Check sheet for the modelled part. Datum: model origin and axes. Units: mm. A direction names the side the tool comes from. Round coordinates to 2 decimals unless told otherwise and drop trailing zeros. Order: outer loops, then holes, each group sorted by start corner. A loop starts at its lowest first (then second) coordinate and runs counter-clockwise, first axis right, second up. Notation, with made-up numbers: (22.25, -40) -> (68.25, -40) arc R22 cw to (68.25, -17) -> close; hole circle Ø11 at (-31.75, 53). An arc over 180 degrees is marked (long way). Use CSV: the item, a comma, the result in double quotes.
```python
from build123d import *

# Parameters (mm, degrees)
BOSS_EXTRUDE1_DEPTH          = 15
SKETCH3_R                    = 40
BOSS_EXTRUDE2_DEPTH          = 100
TAP_DRILL_FOR_M30X2_0_TAP1_D = 28
SKETCH5_R                    = 22.5
CUT_EXTRUDE1_DEPTH           = 50
SKETCH6_W                    = 35
SKETCH6_H                    = 100
BOSS_EXTRUDE3_DEPTH          = 16
SKETCH7_R                    = 15
CUT_EXTRUDE2_DEPTH           = 238.907545067
SKETCH8_W                    = 19
SKETCH8_H                    = 30
SKETCH8_R                    = 5
BOSS_EXTRUDE4_DEPTH          = 77
CUT_EXTRUDE3_DEPTH           = 238.907545067
SKETCH10_R                   = 5
CUT_EXTRUDE4_DEPTH           = 238.907545067
FILLET1_R                    = 1


with BuildPart() as part:
    # Sketch2 → Boss-Extrude1 (new body)
    with BuildSketch(Plane(origin=(0, 0, 0), x_dir=(1, 0, 0), z_dir=(0, 1, 0))):
        with BuildLine():
            Line((-160, 50), (160, 50))
            Line((160, 50), (160, -50))
            Line((160, -50), (-160, -50))
            ThreePointArc((-160, -50), (-210, 0), (-160, 50))
        make_face()
    extrude(amount=BOSS_EXTRUDE1_DEPTH)

    # Sketch3 → Boss-Extrude2 (add)
    with BuildSketch(Plane(origin=(0, 15, 0), x_dir=(1, 0, 0), z_dir=(0, 1, 0))):
        with Locations(Location((-160, 0, 0), (0, 0, 270))):
            Circle(SKETCH3_R)
    extrude(amount=BOSS_EXTRUDE2_DEPTH)

    # Tap Drill for M30x2.0 Tap1 (through all)
    with Locations(Plane(origin=(-160, 115, 0), x_dir=(0, 0, 1), z_dir=(0, 1, 0))):
        with Locations((0, 0)):
            Hole(TAP_DRILL_FOR_M30X2_0_TAP1_D / 2)

    # Sketch5 → Cut-Extrude1 (cut)
    with BuildSketch(Plane(origin=(0, 115, 0), x_dir=(1, 0, 0), z_dir=(0, 1, 0))):
        with Locations(Location((-160, 0, 0), (0, 0, 270))):
            Circle(SKETCH5_R)
    extrude(amount=-CUT_EXTRUDE1_DEPTH, mode=Mode.SUBTRACT)

    # Sketch6 → Boss-Extrude3 (add)
    with BuildSketch(Plane(origin=(0, 15, 0), x_dir=(1, 0, 0), z_dir=(0, 1, 0))):
        with Locations((142.5, 0)):
            Rectangle(SKETCH6_W, SKETCH6_H)
    extrude(amount=BOSS_EXTRUDE3_DEPTH)

    # Sketch7 → Cut-Extrude2 (cut, through all)
    with BuildSketch(Plane(origin=(0, 15, 0), x_dir=(1, 0, 0), z_dir=(0, 1, 0))):
        with Locations(Location((-75, 0, 0), (0, 0, 270))):
            Circle(SKETCH7_R)
    extrude(amount=-CUT_EXTRUDE2_DEPTH, mode=Mode.SUBTRACT)

    # Sketch8 → Boss-Extrude4 (add)
    with BuildSketch(Plane(origin=(0, 15, 0), x_dir=(1, 0, 0), z_dir=(0, 1, 0))):
        with Locations((78, 0)):
            Rectangle(SKETCH8_W, SKETCH8_H)
        with Locations(Location((78, 0, 0), (0, 0, 270))):
            Circle(SKETCH8_R, mode=Mode.SUBTRACT)
    extrude(amount=BOSS_EXTRUDE4_DEPTH)

    # Sketch9 → Cut-Extrude3 (cut, through all)
    with BuildSketch(Plane(origin=(0, 15, 0), x_dir=(1, 0, 0), z_dir=(0, 1, 0))):
        with BuildLine():
            Line((-75, -27.5), (-75, -25))
            ThreePointArc((-75, -25), (-100, 0), (-75, 25))
            Line((-75, 25), (-75, 27.5))
            ThreePointArc((-75, 27.5), (-47.5, 0), (-75, -27.5))
        make_face()
    extrude(amount=-CUT_EXTRUDE3_DEPTH, mode=Mode.SUBTRACT)

    # Sketch10 → Cut-Extrude4 (cut, through all)
    with BuildSketch(Plane(origin=(0, 15, 0), x_dir=(1, 0, 0), z_dir=(0, 1, 0))):
        with Locations(Location((78, 0, 0), (0, 0, 270))):
            Circle(SKETCH10_R)
    extrude(amount=-CUT_EXTRUDE4_DEPTH, mode=Mode.SUBTRACT)

    # Fillet1
    fillet1_edges = [part.edges().sort_by_distance(p)[0] for p in [
        (-160, 65, -22.5),
    ]]
    fillet(fillet1_edges, radius=FILLET1_R)


solid = part.part
```
Q1. Mould release check, pull along Z, two halves, no side actions. Record for faces 1 (the face through (-2, 8, 50)), 2 (the face through (-99.994, 7.605, 0.55)), 3 (the face through (-164, 65, 14)), 4 (the face through (68.5, 53, 0)): pulls with the +Z half, pulls with the -Z half, needs draft (parallel to the pull), parting line crosses it, or undercut.
Result sheet:
face 1,"pulls with the +Z half"
face 2,"undercut"
face 3,"undercut"
face 4,"needs draft"
Q2. Go/stop test with flat-tipped pins: pin 1 (10 mm diameter, centred on y = 93.5, z = 16, fed in from -X); pin 2 (3 mm diameter, centred on y = 36, z = -12, fed in from +X); pin 3 (5 mm diameter, centred on y = 86.5, z = -27, fed in from -X); pin 4 (12 mm diameter, centred on x = 66.5, z = 2, fed in from -Y). Record where each tip stops, or that it passes through.
Result sheet:
pin 1,"stops at x = -198.46"
pin 2,"stops at x = 87.5"
pin 3,"stops at x = -191.62"
pin 4,"stops at y = 0"
Q3. Sectioned sample at A-A, the plane y = 59. Enter the section's corners in (x, z), then the cut area to 3 significant figures.
Result sheet:
outline,"circle Ø80 at (-160, 0); (68.5, -15) -> (87.5, -15) -> (87.5, 15) -> (68.5, 15) -> close; hole circle Ø28 at (-160, 0); hole circle Ø10 at (78, 0)"
area,"4,900 mm^2"
Q4. Sectioned sample at C-C, the plane z = 0. State how many separate pieces and enclosed holes the cut face has, then the cut area to 3 significant figures.
Result sheet:
separate pieces,"4"
enclosed holes,"0"
area,"9,800 mm^2"
Q5. Scan lines: L1, parallel to X at y = 59.5, z = 0; L2, parallel to X at y = 10, z = 0; L3, parallel to X at y = 46, z = -9. Record each from-to range of solid material in increasing order.
Result sheet:
L1,"x = -200 to -174, -146 to -120, 68.5 to 73, 83 to 87.5"
L2,"x = -210 to -174, -146 to -100, -47.5 to 73, 83 to 160"
L3,"x = -198.97 to -170.72, -149.28 to -121.03, 68.5 to 87.5"
Q6. Sectioned sample at D-D, the plane x = 78. Enter the section's corners in (y, z), then the cut area to 3 significant figures.
Result sheet:
outline,"(0, -50) -> (15, -50) -> (15, -15) -> (92, -15) -> (92, -5) -> (0, -5) -> close; (0, 5) -> (92, 5) -> (92, 15) -> (15, 15) -> (15, 50) -> (0, 50) -> close"
area,"2,890 mm^2"
Q7. Sectioned sample at B-B, the plane y = 26.5. Enter the section's corners in (x, z), then the cut area to 3 significant figures.
Result sheet:
outline,"circle Ø80 at (-160, 0); (68.5, -15) -> (87.5, -15) -> (87.5, 15) -> (68.5, 15) -> close; (125, -50) -> (160, -50) -> (160, 50) -> (125, 50) -> close; hole circle Ø28 at (-160, 0); hole circle Ø10 at (78, 0)"
area,"8,400 mm^2"
Q8. Access from +Z, -Z, +X, -X, +Y, -Y to the whole of each face (thin tool, end or side, straight path). Record for faces 5 (the face through (78, 53, -15)), 6 (the face through (-47.507, 7.605, -0.605)), 7 (the face through (82, 92, -4)).
Result sheet:
face 5,"-Z, +Y"
face 6,"+Y, -Y"
face 7,"+Z, -Z, +X, +Y"
